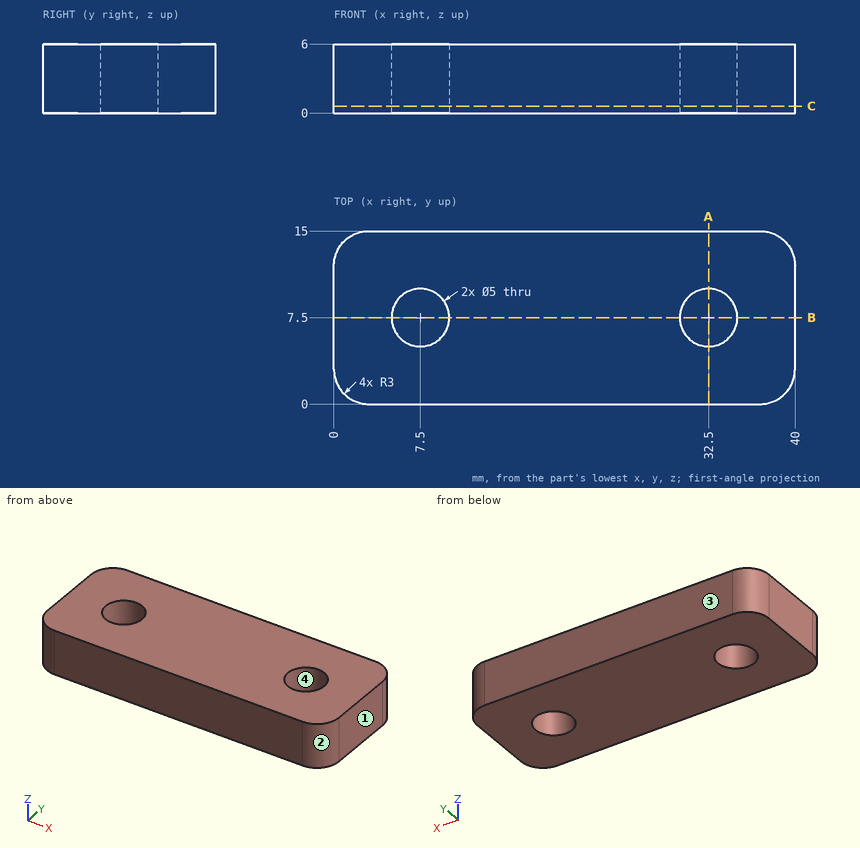
Job drawing, mm, ordinate dimensions from the low corner. One solid piece. Round coordinates to 2 decimals unless told otherwise and drop trailing zeros. Loops run counter-clockwise (first coordinate to the right, second up) from the corner with the lowest first, then second, coordinate; pieces in that order, holes last. Notation, with made-up numbers: (0.25, 39) -> (51.25, 39) arc R24 ccw to (51.25, 59) -> close; hole circle Ø2 at (-11, -12.5). An arc over 180 degrees is marked (long way). Use CSV: the item, a comma, the result in double quotes. Start each with the question number.
Q1. Saw through at A-A on x = 32.5. Give the cut face in (y, z), and give its area (3 significant figures).
Q2. Mould opens along Y. For the marked faces 1, 2, 3 and 4 say: +Y half, -Y half, draft (parallel to the pull), parting line (faces both ways), or undercut.
Q3. Drill centre lines: L1, parallel to X at y = 8, z = 2.9; L2, parallel to X at y = 6.25, z = 2.55; L3, parallel to Y at x = 32.5, z = 4.4. Where is each one in solid material? Low to high.
Q4. Flat gauge pins, fed straight in: pin 1 Ø3 at (x, y) = (7.5, 7.5) entering from -Z; pin 2 Ø2 at (x, z) = (34.5, 2) entering from -Y. Where does each tip first touch, or does it go through?
Q5. Saw through at B-B on y = 7.5. Give the cut face in (x, z), and give its area (3 significant figures).
Q6. Saw through at C-C on z = 0.6. Give the cut face in (x, y).
Solutions:
1,outline,"(0, 0) -> (5, 0) -> (5, 6) -> (0, 6) -> close; (10, 0) -> (15, 0) -> (15, 6) -> (10, 6) -> close"
1,area,"60.0 mm^2"
2,face 1,"draft"
2,face 2,"-Y half"
2,face 3,"+Y half"
2,face 4,"undercut"
3,L1,"x = 0 to 5.05, 9.95 to 30.05, 34.95 to 40"
3,L2,"x = 0 to 5.33, 9.67 to 30.33, 34.67 to 40"
3,L3,"y = 0 to 5, 10 to 15"
4,pin 1,"passes through"
4,pin 2,"stops at y = 0"
5,outline,"(0, 0) -> (5, 0) -> (5, 6) -> (0, 6) -> close; (10, 0) -> (30, 0) -> (30, 6) -> (10, 6) -> close; (35, 0) -> (40, 0) -> (40, 6) -> (35, 6) -> close"
5,area,"180 mm^2"
6,outline,"(0, 3) arc R3 ccw to (3, 0) -> (37, 0) arc R3 ccw to (40, 3) -> (40, 12) arc R3 ccw to (37, 15) -> (3, 15) arc R3 ccw to (0, 12) -> close; hole circle Ø5 at (7.5, 7.5); hole circle Ø5 at (32.5, 7.5)"
